For this review, take the finished solid that the model builds, in its own axes (mm). A direction names the side the tool comes from. Give positions to 0.01 mm unless a question says otherwise; leave off trailing zeros. Write each loop counter-clockwise with the first axis right and the second up, starting at its lowest first coordinate (ties: lowest second). Pieces come first, ordered by that corner, then holes.
1) Wall thickness on line 1 along X through (y, z) = (-0.7, -8); line 2 along Y through (x, z) = (4, 11.5); line 3 along X through (y, z) = (9, -10.25): over which ranges is each line inside the solid? List them lowest first.
2) Machinability: for faces 4 (the face through (1, 0, -6)), 5 (the face through (-14.99, 27.591, 9.293)), which of the approach directions +Z, -Z, +X, -X, +Y, -Y give a long, thin tool a straight path to every point of the face, cutting with its end or side? Answer none if there is none.
3) For P1, Ø8, axis at y = 9, z = -5, coming from the +X side; P2, Ø8, axis at x = 2, y = 6, coming from the -Z side; P3, Ø6.5, axis at x = -7.35, z = -8, coming from the +Y side, all flat-tipped, find the tip position at first contact; note any pin that passes through.
4) We need section B-B on x = 0.65. Give the boundary of the cut face in (y, z).
5) We need section C-C on z = 8. Give the boundary of the cut face in (x, y).
6) We need section A-A on x = 8.65. Give the boundary of the cut face in (y, z), and give its area (3 significant figures).
7) Draft analysis for pull direction X (two halves, no side actions). For faces 1 (the face through (-15.75, 11, 0)), 2 (the face through (15.75, -1, 0)), 3 (the face through (4.866, -0.74, 2.688)), state which applies: pulls with the +X half, pulls with the -X half, needs draft (parallel to the pull), parting line crosses it, or undercut.
8) We need section D-D on y = 20. Give the boundary of the cut face in (x, z), and give its area (3 significant figures).
from build123d import *

# Parameters (mm, degrees)
SKETCH3_W           = 31.5
SKETCH3_H           = 26
BOSS_EXTRUDE1_DEPTH = 1.5
SKETCH4_W           = 1.5
SKETCH4_H           = 26
BOSS_EXTRUDE3_DEPTH = 31.5
FILLET3_R           = 13
FILLET4_R           = 13
SKETCH5_R           = 4
CUT_EXTRUDE1_DEPTH  = 31.5
SKETCH7_R           = 2
SKETCH7_R_2         = 5
CUT_EXTRUDE2_DEPTH  = 10


with BuildPart() as part:
    # Sketch3 → Boss-Extrude1 (new body)
    with BuildSketch(Plane(origin=(0, 0, 0), x_dir=(1, 0, 0), z_dir=(0, 1, 0))):
        Rectangle(SKETCH3_W, SKETCH3_H)
    extrude(amount=-BOSS_EXTRUDE1_DEPTH)

    # Sketch4 → Boss-Extrude3 (add)
    with BuildSketch(Plane(origin=(0, 0, 0), x_dir=(1, 0, 0), z_dir=(0, 1, 0))):
        with Locations((-15, 0)):
            Rectangle(SKETCH4_W, SKETCH4_H)
    extrude(amount=BOSS_EXTRUDE3_DEPTH)

    # Fillet3
    fillet3_edges = [part.edges().sort_by_distance(p)[0] for p in [
        (-15, 31.5, 13),
    ]]
    fillet(fillet3_edges, radius=FILLET3_R)

    # Fillet4
    fillet4_edges = [part.edges().sort_by_distance(p)[0] for p in [
        (-15, 31.5, -13),
    ]]
    fillet(fillet4_edges, radius=FILLET4_R - 0.0001)  # a hair under: the kernel refuses the full size

    # Sketch5 → Cut-Extrude1 (cut)
    with BuildSketch(Plane(origin=(-14.25, 0, 0), x_dir=(0, 0, -1), z_dir=(1, 0, 0))):
        with Locations((0, 18.5)):
            Circle(SKETCH5_R)
    extrude(amount=-CUT_EXTRUDE1_DEPTH, mode=Mode.SUBTRACT)

    # Sketch7 → Cut-Extrude2 (cut)
    with BuildSketch(Plane(origin=(0, 0, 0), x_dir=(1, 0, 0), z_dir=(0, 1, 0))):
        with Locations(Location((8.65, 8, 0), (0, 0, 270))):
            Circle(SKETCH7_R)
        with Locations(Location((8.65, -8, 0), (0, 0, 270))):
            Circle(SKETCH7_R)
        with Locations(Location((0.65, 0, 0), (0, 0, 270))):
            Circle(SKETCH7_R_2)
        with Locations(Location((-7.35, 8, 0), (0, 0, 270))):
            Circle(SKETCH7_R)
        with Locations(Location((-7.35, -8, 0), (0, 0, 270))):
            Circle(SKETCH7_R)
    extrude(amount=-CUT_EXTRUDE2_DEPTH, mode=Mode.SUBTRACT)


solid = part.part
Results list:
1. line 1: x = -15.75 to -9.35, -5.35 to 6.65, 10.65 to 15.75
1. line 2: y = -1.5 to 0
1. line 3: x = -15.75 to -14.25
2. face 4: +Z, -Z, +X, +Y
2. face 5: +Z, +X, -X, +Y
3. P1: stops at x = -14.25
3. P2: passes through
3. P3: stops at y = 0
4. outline: (-1.5, -13) - (0, -13) - (0, -5) - (-1.5, -5) - close; (-1.5, 5) - (0, 5) - (0, 13) - (-1.5, 13) - close
5. outline: (-15.75, -1.5) - (-9.35, -1.5) - (-9.35, 0) - (-14.25, 0) - (-14.25, 28.75) - (-15.75, 28.75) - close; (-5.35, -1.5) - (6.65, -1.5) - (6.65, 0) - (-5.35, 0) - close; (10.65, -1.5) - (15.75, -1.5) - (15.75, 0) - (10.65, 0) - close
6. outline: (-1.5, -13) - (0, -13) - (0, -10) - (-1.5, -10) - close; (-1.5, -6) - (0, -6) - (0, 6) - (-1.5, 6) - close; (-1.5, 10) - (0, 10) - (0, 13) - (-1.5, 13) - close
6. area: 27.0 mm2
7. face 1: pulls with the -X half
7. face 2: pulls with the +X half
7. face 3: undercut
8. outline: (-15.75, -12.91) - (-14.25, -12.91) - (-14.25, -3.71) - (-15.75, -3.71) - close; (-15.75, 3.71) - (-14.25, 3.71) - (-14.25, 12.91) - (-15.75, 12.91) - close
8. area: 27.6 mm2
